Part model, mm, in its own coordinate system. Round coordinates to 2 decimals unless told otherwise and drop trailing zeros. Write each loop counter-clockwise with the first axis right and the second up, starting at its lowest first coordinate (ties: lowest second). Pieces come first, ordered by that corner, then holes. Notation, with made-up numbers: (53.5, -3) -> (77.5, -3) arc R21 ccw to (77.5, 27) -> close; hole circle Ø9 at (83.25, 32). An arc over 180 degrees is marked (long way). Return JSON: item names as keys, results as strings. Group by question number.
(1) Drop flat-ended pins along their axis: pin 1 Ø3 at (y, z) = (3.5, -20.5) entering from +X; pin 2 Ø1 at (y, z) = (3.5, 64.5) entering from +X; pin 3 Ø1 at (y, z) = (5, -69) entering from +X. Give the stop position or say it passes through.
(2) Drill centre lines: L1, parallel to Z at x = 72, y = 6.5; L2, parallel to Z at x = -36, y = 4.5; L3, parallel to X at y = 3.75, z = 0. Where is each one in solid material? Low to high. Write a range as from..to.
(3) Saw through at C-C (y = 4). State how many separate pieces and enclosed holes the cut face has, plus the area to 3 significant figures.
(4) Saw through at A-A (x = 44.5). List the corners of the cut face in (y, z), plus the area to 3 significant figures.
(5) Saw through at B-B (z = 34). List the corners of the cut face in (x, y).
from build123d import *

# Parameters (mm, degrees)
SKETCH_1_R          = 100
EXTRUDE_2_DEPTH     = 8
SKETCH_3_R          = 5
SKETCH_3_R_2        = 1.5
CUT_EXTRUDE_1_DEPTH = 142.647449677
FILLET_1_R          = 7
FILLET_2_R          = 7


with BuildPart() as part:
    # 草图1 → 凸台-拉伸2 (new body)
    with BuildSketch(Plane(origin=(0, 0, 0), x_dir=(1, 0, 0), z_dir=(0, 1, 0))):
        with Locations(Location((0, 0, 0), (0, 0, 270))):
            Circle(SKETCH_1_R)
        with BuildLine():
            Line((-22.971939134, 87.411215106), (-9.292268133, 20.49155321))
            ThreePointArc((-9.292268133, 20.49155321), (-21.343901201, 7.119542226), (-19.733222484, -10.809714631))
            Line((-19.733222484, -10.809714631), (-70.847514199, -56.116488181))
            ThreePointArc((-70.847514199, -56.116488181), (-85.735481912, 28.5982107), (-22.971939134, 87.411215106))
        make_face(mode=Mode.SUBTRACT)
        with BuildLine():
            Line((-13.174547237, 89.413991181), (0.505123764, 22.494329285))
            ThreePointArc((0.505123764, 22.494329285), (16.837655032, 14.924589543), (22.392339709, -2.198436343))
            Line((22.392339709, -2.198436343), (87.186302424, -23.811324689))
            ThreePointArc((87.186302424, -23.811324689), (67.634517925, 59.949999991), (-13.174547237, 89.413991181))
        make_face(mode=Mode.SUBTRACT)
        with BuildLine():
            Line((19.22809872, -11.684614654), (84.022061435, -33.297503))
            ThreePointArc((84.022061435, -33.297503), (18.100963986, -88.548210691), (-64.21436329, -63.599890417))
            Line((-64.21436329, -63.599890417), (-13.100071576, -18.293116867))
            ThreePointArc((-13.100071576, -18.293116867), (4.50624617, -22.044131769), (19.22809872, -11.684614654))
        make_face(mode=Mode.SUBTRACT)
    extrude(amount=EXTRUDE_2_DEPTH)

    # 草图3 → 切除-拉伸1 (cut, through all)
    with BuildSketch(Plane(origin=(0, 8, 0), x_dir=(1, 0, 0), z_dir=(0, 1, 0))):
        with Locations(Location((0, 0, 0), (0, 0, 270))):
            Circle(SKETCH_3_R)
        with Locations(Location((-3.104302917, 15.185957441, 0), (0, 0, 270))):
            Circle(SKETCH_3_R_2)
        with Locations(Location((15.185957441, 3.104302917, 0), (0, 0, 270))):
            Circle(SKETCH_3_R_2)
        with Locations(Location((3.104302917, -15.185957441, 0), (0, 0, 270))):
            Circle(SKETCH_3_R_2)
        with Locations(Location((-15.185957441, -3.104302917, 0), (0, 0, 270))):
            Circle(SKETCH_3_R_2)
    extrude(amount=-CUT_EXTRUDE_1_DEPTH, mode=Mode.SUBTRACT)

    # 圆角1
    fillet_1_edges = [part.edges().sort_by_distance(p)[0] for p in [
        (87.186302424, 4, 23.811324689),
        (-13.174547237, 4, -89.413991181),
        (-64.21436329, 4, 63.599890417),
        (84.022061435, 4, 33.297503),
        (-22.971939134, 4, -87.411215106),
        (-70.847514199, 4, 56.116488181),
    ]]
    fillet(fillet_1_edges, radius=FILLET_1_R)

    # 圆角2
    fillet_2_edges = [part.edges().sort_by_distance(p)[0] for p in [
        (0.505123764, 4, -22.494329285),
        (22.392339709, 4, 2.198436343),
        (19.22809872, 4, 11.684614654),
        (-13.100071576, 4, 18.293116867),
        (-19.733222484, 4, 10.809714631),
        (-9.292268133, 4, -20.49155321),
    ]]
    fillet(fillet_2_edges, radius=FILLET_2_R)


solid = part.part
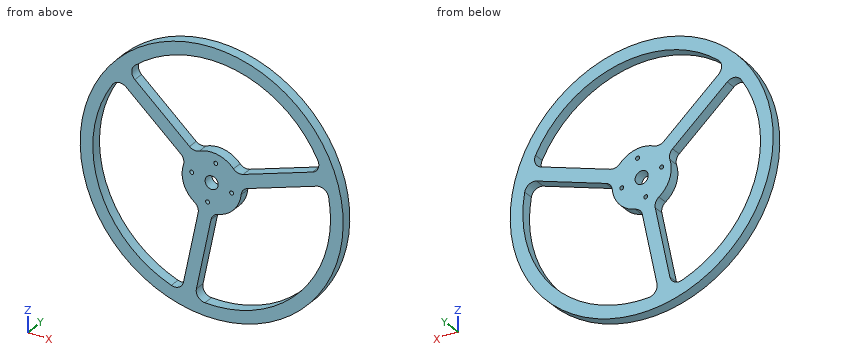
Computed values:
{
 "1": {"pin 1": "x = 98.18", "pin 2": "x = 76.84", "pin 3": "x = 72.85"},
 "2": {"L1": "-69.4..-54.63, 18.75..29.29, 54.63..69.4", "L2": "-93.3..-82.9, 25.23..38.59, 82.9..93.3", "L3": "-100..-90.38, -22.5..-5, 5..22.97, 90.38..100"},
 "3": {"separate pieces": "1", "enclosed holes": "8", "area": "9,390 mm2"},
 "4": {"outline": "(0, -89.55) -> (8, -89.55) -> (8, -78.66) -> (0, -78.66) -> close; (0, 9.57) -> (8, 9.57) -> (8, 20.11) -> (0, 20.11) -> close; (0, 78.66) -> (8, 78.66) -> (8, 89.55) -> (0, 89.55) -> close", "area": "259 mm2"},
 "5": {"outline": "(-94.04, 0) -> (-83.74, 0) -> (-83.74, 8) -> (-94.04, 8) -> close; (-45.9, 0) -> (-30.82, 0) -> (-30.82, 8) -> (-45.9, 8) -> close; (80.54, 0) -> (94.04, 0) -> (94.04, 8) -> (80.54, 8) -> close"}
}
